Could you check a few things on this drawing? It's one solid part, dimensions in mm from its lowest x, y, z. Round coordinates to 2 decimals unless told otherwise and drop trailing zeros. Loops run counter-clockwise (first coordinate to the right, second up) from the corner with the lowest first, then second, coordinate; pieces in that order, holes last. Notation, with made-up numbers: M 40.5,-27.75 L 65.5,-27.75 A14 cw 65.5,-21.75 Z; hole C 18,-0.75 d2. An arc over 180 degrees is marked long. Put each result on its own line as item: value. Start each with the question number.
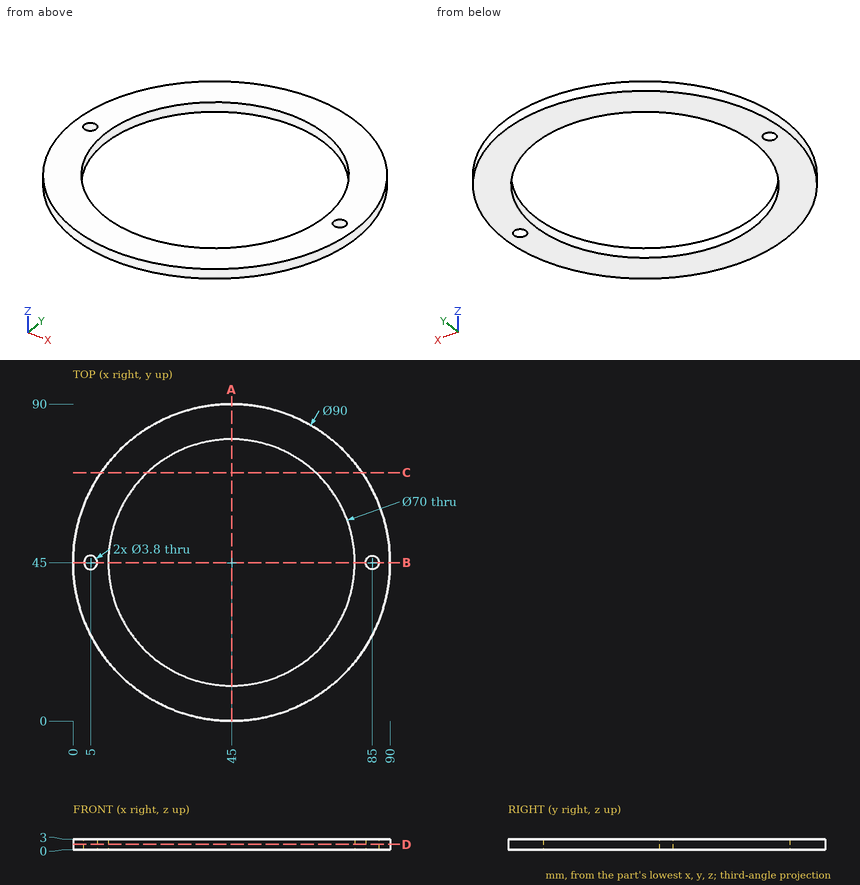
1) I'm going to push flat-ended pins straight in: P1, Ø1, axis at y = 46.5, z = 2.5, coming from the -X side; P2, Ø1, axis at x = 28.5, z = 2.5, coming from the +Y side. Where does each tip first touch, or does it pass through?
2) Suppose I cut it at D-D (z = 1.5). Write out the boundary of the cut face in (x, y), plus the area to 3 significant figures.
3) Suppose I cut it at C-C (y = 70.5). Write out the boundary of the cut face in (x, z).
4) If I drill on probe 1 along Y at (x, z) = (18.5, 1.45); probe 2 along Y at (x, z) = (45, 1.2); probe 3 along X at (y, z) = (33, 1), over which ranges is the centre line in solid material (lowest first)? Write a range as from..to.
5) Suppose I cut it at B-B (y = 45). Write out the boundary of the cut face in (x, z).
6) Suppose I cut it at A-A (x = 45). Write out the boundary of the cut face in (y, z).
Results are:
1. P1: x = 0.01
1. P2: y = 87.06
2. outline: C 45,45 d90; hole C 5,45 d3.8; hole C 45,45 d70; hole C 85,45 d3.8
2. area: 2,490 mm²
3. outline: M 7.92,0 L 21.03,0 L 21.03,3 L 7.92,3 Z; M 68.97,0 L 82.08,0 L 82.08,3 L 68.97,3 Z
4. probe 1: 8.63..22.14, 67.86..81.37
4. probe 2: 0..10, 80..90
4. probe 3: 1.63..12.12, 77.88..88.37
5. outline: M 0,0 L 3.1,0 L 3.1,3 L 0,3 Z; M 6.9,0 L 10,0 L 10,3 L 6.9,3 Z; M 80,0 L 83.1,0 L 83.1,3 L 80,3 Z; M 86.9,0 L 90,0 L 90,3 L 86.9,3 Z
6. outline: M 0,0 L 10,0 L 10,3 L 0,3 Z; M 80,0 L 90,0 L 90,3 L 80,3 Z
